Here's how the part is built. I have some questions about the finished solid (model axes, mm). A direction names the side the tool comes from. Give positions to 0.01 mm unless a question says otherwise; leave off trailing zeros. Loops run counter-clockwise (first coordinate to the right, second up) from the corner with the lowest first, then second, coordinate; pieces in that order, holes last. Notation, with made-up numbers: (81.5, 2.25) -> (139.5, 2.25) arc R25 cw to (139.5, 28.25) -> close; hole circle Ø8 at (61.25, 1.25). An arc over 180 degrees is marked (long way). Answer in a Markdown table with one row per item. Add a question column.
Item 1: If we section it at B-B (x = -91.5): Write out the boundary of the cut face in (y, z), then the cut area to 3 significant figures.
Item 2: If we section it at C-C (z = -21.5): Write out the boundary of the cut face in (x, y), then the cut area to 3 significant figures.
Item 3: If I drill on line 1 (X direction, y = 4, z = 15); line 2 (X direction, y = 1.5, z = -68); line 3 (Z direction, x = -111, y = 1), over which ranges is the centre line in solid material (lowest first)?
Item 4: Which directions (+Z, -Z, +X, -X, +Y, -Y) give clear straight access to the entire face, cutting with the end or side of a thin tool? Please do faces 1 (the face through (0, 3, 11)), 2 (the face through (-120, 3, 11)).
Item 5: If we section it at A-A (y = 1.5): Write out the boundary of the cut face in (x, z), then the cut area to 3 significant figures.
Item 6: For P1, Ø3, axis at y = 3, z = 13, coming from the +X side, with a flat end and sliding along its axis, tell me the tip position at first contact or that it passes through.
```python
from build123d import *

# Parameters (mm, degrees)
BOSS_EXTRUDE1_DEPTH = 6.35
SKETCH3_W           = 120
SKETCH3_H           = 21.5
BOSS_EXTRUDE2_DEPTH = 6.35


with BuildPart() as part:
    # Sketch1 → Boss-Extrude1 (new body)
    with BuildSketch(Plane(origin=(0, 0, 0), x_dir=(1, 0, 0), z_dir=(0, 1, 0))):
        Polygon((-120, 0), (0, 0), (17, 88), (-44, 88), align=None)
    extrude(amount=BOSS_EXTRUDE1_DEPTH)

    # Sketch3 → Boss-Extrude2 (add)
    with BuildSketch(Plane(origin=(0, 0, 0), x_dir=(1, 0, 0), z_dir=(0, 1, 0))):
        with Locations((-60, -10.75)):
            Rectangle(SKETCH3_W, SKETCH3_H)
    extrude(amount=BOSS_EXTRUDE2_DEPTH)


solid = part.part
```
Recorded:
| question | item | result |
|---|---|---|
| 1 | outline | (0, -33) -> (6.35, -33) -> (6.35, 21.5) -> (0, 21.5) -> close |
| 1 | area | 346 mm^2 |
| 2 | outline | (-101.43, 0) -> (4.15, 0) -> (4.15, 6.35) -> (-101.43, 6.35) -> close |
| 2 | area | 670 mm^2 |
| 3 | line 1 | x = -120 to 0 |
| 3 | line 2 | x = -61.27 to 13.14 |
| 3 | line 3 | z = -10.42 to 21.5 |
| 4 | face 1 | +Z, +X, +Y, -Y |
| 4 | face 2 | +Z, -Z, -X, +Y, -Y |
| 5 | outline | (-120, 0) -> (-44, -88) -> (17, -88) -> (0, 0) -> (0, 21.5) -> (-120, 21.5) -> close |
| 5 | area | 10,500 mm^2 |
| 6 | P1 | stops at x = 0 |
